```python
from build123d import *

# Parameters (mm, degrees)
SKETCH1_W                      = 182.88
SKETCH1_H                      = 66.04
BOSS_EXTRUDE2_DEPTH            = 5.08
FILLET2_R                      = 12.7
CUT_EXTRUDE1_DEPTH             = 195.504967546
CUT_EXTRUDE1_DEPTH_BACK        = 195.504967546
SKETCH3_R                      = 3.175
BOSS_EXTRUDE6_DEPTH            = 30.48
SKETCH7_W                      = 10.16
SKETCH7_H                      = 10.16
BOSS_EXTRUDE8_DEPTH            = 5.08
SKETCH10_R                     = 1.27
BOSS_EXTRUDE10_DEPTH           = 2.54
CUT_EXTRUDE4_REACH             = 199.664
SKETCH12_W                     = 10.16
SKETCH12_H                     = 10.16
CUT_EXTRUDE4_DIRECTION_2_DEPTH = 198.663576817
CUT_EXTRUDE5_REACH             = 199.664
SKETCH14_W                     = 10.16
SKETCH14_H                     = 10.16
FILLET5_R                      = 2.032
FILLET6_R                      = 5.08
FILLET7_R                      = 2.54


with BuildPart() as part:
    # Sketch1 → Boss-Extrude2 (new body)
    with BuildSketch(Plane(origin=(0, 0, 0), x_dir=(1, 0, 0), z_dir=(0, 1, 0))):
        with Locations((-91.44, 33.02)):
            Rectangle(SKETCH1_W, SKETCH1_H)
    extrude(amount=BOSS_EXTRUDE2_DEPTH)

    # Fillet2
    fillet2_edges = [part.edges().sort_by_distance(p)[0] for p in [
        (0, 2.54, 0),
        (-182.88, 2.54, 0),
        (-182.88, 2.54, -66.04),
        (0, 2.54, -66.04),
    ]]
    fillet(fillet2_edges, radius=FILLET2_R)

    # Sketch3 → Cut-Extrude1 (cut, two sides: drawn at the far end of the back side and taken through both)
    with BuildSketch(Plane(origin=(0, 5.08, 0), x_dir=(1, 0, 0), z_dir=(0, 1, 0)).offset(-CUT_EXTRUDE1_DEPTH_BACK)):
        with Locations(Location((-12.7, 12.7, 0), (0, 0, 270))):
            Circle(SKETCH3_R)
        with Locations(Location((-12.7, 53.34, 0), (0, 0, 270))):
            Circle(SKETCH3_R)
        with Locations(Location((-170.18, 53.34, 0), (0, 0, 270))):
            Circle(SKETCH3_R)
        with Locations(Location((-170.18, 12.7, 0), (0, 0, 270))):
            Circle(SKETCH3_R)
    extrude(amount=CUT_EXTRUDE1_DEPTH + CUT_EXTRUDE1_DEPTH_BACK, mode=Mode.SUBTRACT)

    # Sketch4 → Boss-Extrude6 (add)
    with BuildSketch(Plane(origin=(0, 5.08, 0), x_dir=(1, 0, 0), z_dir=(0, 1, 0))):
        Polygon((-157.48, 0), (-30.606358486, 0), (-25.4, 0), (-25.4, 66.04), (-157.48, 66.04), align=None)
        Polygon((-27.94, 55.88), (-27.94, 10.16), (-27.94, 2.54), (-35.56, 2.54), (-147.32, 2.54), (-154.94, 2.54), (-154.94, 10.16), (-154.94, 55.88), (-154.94, 63.5), (-147.32, 63.5), (-35.56, 63.5), (-27.94, 63.5), align=None, mode=Mode.SUBTRACT)
    extrude(amount=BOSS_EXTRUDE6_DEPTH)

    # Sketch7 → Boss-Extrude8 (add)
    with BuildSketch(Plane(origin=(0, 5.08, 0), x_dir=(1, 0, 0), z_dir=(0, 1, 0))):
        with Locations((-33.02, 7.62)):
            Rectangle(SKETCH7_W, SKETCH7_H)
        with Locations((-149.86, 7.62)):
            Rectangle(SKETCH7_W, SKETCH7_H)
        with Locations((-149.86, 58.42)):
            Rectangle(SKETCH7_W, SKETCH7_H)
        with Locations((-33.02, 58.42)):
            Rectangle(SKETCH7_W, SKETCH7_H)
    extrude(amount=BOSS_EXTRUDE8_DEPTH)

    # Sketch10 → Boss-Extrude10 (add)
    with BuildSketch(Plane(origin=(0, 10.16, 0), x_dir=(1, 0, 0), z_dir=(0, 1, 0))):
        with Locations(Location((-34.544, 9.144, 0), (0, 0, 270))):
            Circle(SKETCH10_R)
        with Locations(Location((-148.336, 9.144, 0), (0, 0, 270))):
            Circle(SKETCH10_R)
        with Locations(Location((-148.336, 56.896, 0), (0, 0, 270))):
            Circle(SKETCH10_R)
        with Locations(Location((-34.544, 56.896, 0), (0, 0, 270))):
            Circle(SKETCH10_R)
    extrude(amount=BOSS_EXTRUDE10_DEPTH)

    # Sketch12 → Cut-Extrude4 (cut, up to next)
    with BuildSketch(Plane(origin=(0, 0, -66.04), x_dir=(-1, 0, 0), z_dir=(0, 0, -1)), mode=Mode.PRIVATE) as cut_extrude4_sk1:
        with Locations((38.1, 15.24)):
            Rectangle(SKETCH12_W, SKETCH12_H)
    cut_extrude4_tool1 = extrude(cut_extrude4_sk1.sketch, amount=-CUT_EXTRUDE4_REACH, mode=Mode.PRIVATE) & part.part
    # Sketch12 → Cut-Extrude4 (cut, up to next)
    with BuildSketch(Plane(origin=(0, 0, -66.04), x_dir=(-1, 0, 0), z_dir=(0, 0, -1)), mode=Mode.PRIVATE) as cut_extrude4_sk2:
        with Locations((60.96, 15.24)):
            Rectangle(SKETCH12_W, SKETCH12_H)
    cut_extrude4_tool2 = extrude(cut_extrude4_sk2.sketch, amount=-CUT_EXTRUDE4_REACH, mode=Mode.PRIVATE) & part.part
    add(cut_extrude4_tool1.solids().sort_by_distance((-38.1, 15.24, -66.04))[0], mode=Mode.SUBTRACT)
    add(cut_extrude4_tool2.solids().sort_by_distance((-60.96, 15.24, -66.04))[0], mode=Mode.SUBTRACT)

    # Sketch12 → Cut-Extrude4 direction 2 (cut)
    with BuildSketch(Plane(origin=(0, 0, -66.04), x_dir=(-1, 0, 0), z_dir=(0, 0, -1))):
        with Locations((38.1, 15.24)):
            Rectangle(SKETCH12_W, SKETCH12_H)
        with Locations((60.96, 15.24)):
            Rectangle(SKETCH12_W, SKETCH12_H)
    extrude(amount=CUT_EXTRUDE4_DIRECTION_2_DEPTH, mode=Mode.SUBTRACT)

    # Sketch14 → Cut-Extrude5 (cut, up to next)
    with BuildSketch(Plane.XY, mode=Mode.PRIVATE) as cut_extrude5_sk1:
        with Locations((-38.1, 15.24)):
            Rectangle(SKETCH14_W, SKETCH14_H)
    cut_extrude5_tool1 = extrude(cut_extrude5_sk1.sketch, amount=-CUT_EXTRUDE5_REACH, mode=Mode.PRIVATE) & part.part
    # Sketch14 → Cut-Extrude5 (cut, up to next)
    with BuildSketch(Plane.XY, mode=Mode.PRIVATE) as cut_extrude5_sk2:
        with Locations((-60.96, 15.24)):
            Rectangle(SKETCH14_W, SKETCH14_H)
    cut_extrude5_tool2 = extrude(cut_extrude5_sk2.sketch, amount=-CUT_EXTRUDE5_REACH, mode=Mode.PRIVATE) & part.part
    add(cut_extrude5_tool1.solids().sort_by_distance((-38.1, 15.24, 0))[0], mode=Mode.SUBTRACT)
    add(cut_extrude5_tool2.solids().sort_by_distance((-60.96, 15.24, 0))[0], mode=Mode.SUBTRACT)

    # Fillet5
    fillet5_edges = [part.edges().sort_by_distance(p)[0] for p in [
        (-33.02, 20.32, -64.77),
        (-33.02, 10.16, -64.77),
        (-43.18, 10.16, -64.77),
        (-43.18, 20.32, -64.77),
        (-55.88, 20.32, -64.77),
        (-55.88, 10.16, -64.77),
        (-66.04, 10.16, -64.77),
        (-66.04, 20.32, -64.77),
        (-43.18, 20.32, -1.27),
        (-33.02, 20.32, -1.27),
        (-33.02, 10.16, -1.27),
        (-66.04, 10.16, -1.27),
        (-66.04, 20.32, -1.27),
        (-55.88, 20.32, -1.27),
        (-55.88, 10.16, -1.27),
    ]]
    fillet(fillet5_edges, radius=FILLET5_R)

    # Fillet6
    fillet6_edges = [part.edges().sort_by_distance(p)[0] for p in [
        (-157.48, 20.32, -66.04),
        (-157.48, 20.32, 0),
        (-25.4, 20.32, 0),
        (-25.4, 20.32, -66.04),
    ]]
    fillet(fillet6_edges, radius=FILLET6_R)

    # Fillet7
    fillet7_edges = [part.edges().sort_by_distance(p)[0] for p in [
        (-27.94, 22.86, -2.54),
        (-154.94, 22.86, -2.54),
        (-154.94, 22.86, -63.5),
        (-27.94, 22.86, -63.5),
    ]]
    fillet(fillet7_edges, radius=FILLET7_R)


solid = part.part
```
Can you work these out from the model? Positions are in its coordinate system, mm. A direction names the side the tool comes from. Give positions to 0.01 mm unless a question says otherwise; leave off trailing zeros. Order: outer loops, then holes, each group sorted by start corner. A loop starts at its lowest first (then second) coordinate and runs counter-clockwise, first axis right, second up. Notation, with made-up numbers: M 75,-10 L 81,-10 A26 cw 81,14 Z; hole C 20,79 d3. An arc over 180 degrees is marked long. Write item = value, one per line. Start each with the question number.
Q1. Suppose I cut it at D-D (x = -160). Write out the boundary of the cut face in (y, z), plus the area to 3 significant figures.
Q2. I need wall thicknesses on probe 1 along X at (y, z) = (2.8, -53.34) (3 decimals); probe 2 along X at (y, z) = (1, -53); probe 3 along Z at (x, y) = (-118, 30.5). Which ranges of each line are inside material? Lowest first, please. Write a range as [from, to].
Q3. For faces 4 (the cylindrical face through (-155.952, 20.533, -64.591)), 5 (the flat face through (-25.4, 20, -33)), 6 (the cylindrical face through (-179.26, 2.58, -62.22)), 7 (the flat face through (-38.1, 8, -8)), which set-ups out of +Z, -Z, +X, -X, +Y, -Y let a thin tool reach every point of the face, with its end or its side?
Q4. We'd pull the mould along Y, two halves only. Please class faces 1 (the flat face through (-144.78, 8, -8)), 2 (the flat face through (-150, 10.16, -58)), 3 (the flat face through (-33, 10.16, -60)): pulls with the +Y half, pulls with the -Y half, needs draft (parallel to the pull), parting line crosses it, or undercut.
Q5. Suppose I cut it at B-B (y = 27). Write out the boundary of the cut face in (x, z).
Q6. Will these pins go through, and if not, where does the flat tip stop? pin 1 Ø2 at (x, z) = (-148.5, -9) entering from +Y; pin 2 Ø2 at (y, z) = (14.5, -65) entering from -X; pin 3 Ø8 at (x, z) = (-43.5, -48) entering from +Y.
Q7. Suppose I cut it at C-C (x = -86). Write out the boundary of the cut face in (y, z).
Q8. Suppose I cut it at A-A (z = -43.5). Write out the boundary of the cut face in (x, y), plus the area to 3 significant figures.
Check result:
q1.outline = M 0,-66.04 L 5.08,-66.04 L 5.08,0 L 0,0 Z
q1.area = 335 mm2
q2.probe_1 = [-182.88, -173.355], [-167.005, -15.875], [-9.525, 0]
q2.probe_2 = [-182.88, -173.34], [-167.02, -15.86], [-9.54, 0]
q2.probe_3 = [-66.04, -63.5], [-2.54, 0]
q3.face_4 = -Z, -X, +Y
q3.face_5 = +Z, -Z, +X, +Y
q3.face_6 = -Z, -X, +Y, -Y
q3.face_7 = +Y
q4.face_1 = needs draft
q4.face_2 = pulls with the +Y half
q4.face_3 = undercut
q5.outline = M -157.48,-60.96 A5.08 ccw -152.4,-66.04 L -30.48,-66.04 A5.08 ccw -25.4,-60.96 L -25.4,-5.08 A5.08 ccw -30.48,0 L -152.4,0 A5.08 ccw -157.48,-5.08 Z; hole M -154.94,-60.96 A2.54 ccw -152.4,-63.5 L -30.48,-63.5 A2.54 ccw -27.94,-60.96 L -27.94,-5.08 A2.54 ccw -30.48,-2.54 L -152.4,-2.54 A2.54 ccw -154.94,-5.08 Z
q6.pin_1 = 12.7
q6.pin_2 = -156.47
q6.pin_3 = 5.08
q7.outline = M 0,-66.04 L 35.56,-66.04 L 35.56,-63.5 L 5.08,-63.5 L 5.08,-2.54 L 35.56,-2.54 L 35.56,0 L 0,0 Z
q8.outline = M -182.88,0 L 0,0 L 0,5.08 L -25.4,5.08 L -25.4,35.56 L -27.94,35.56 L -27.94,5.08 L -154.94,5.08 L -154.94,35.56 L -157.48,35.56 L -157.48,5.08 L -182.88,5.08 Z
q8.area = 1,080 mm2
